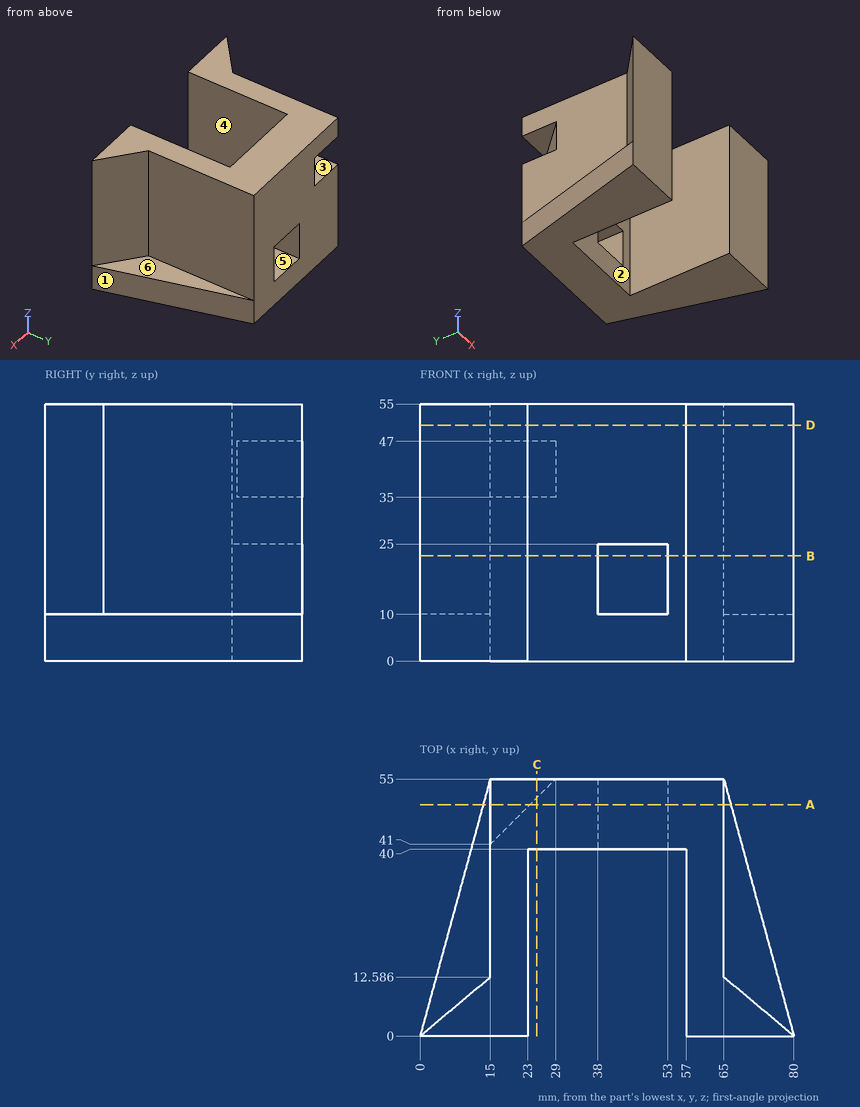
Design review of the part shown in the three views and the two pictorial views. Dimensions are in mm from the part's minimum x, y and z. A direction names the side the tool comes from. Give positions to 0.01 mm unless a question says otherwise; leave off trailing zeros. Loops run counter-clockwise (first coordinate to the right, second up) from the corner with the lowest first, then second, coordinate; pieces in that order, holes last. Notation, with made-up numbers: (61, -28) -> (116, -28) arc R17 cw to (116, -10) -> close; hole circle Ø3 at (78, 22.25). An arc over 180 degrees is marked (long way). Write each question's results on one line, items separated by ' | '.
1) Take a section at D-D, the plane z = 50.5. Give the boundary of the cut face in (x, y), plus the area to 3 significant figures.
Conclusion:
outline: (0, 0) -> (23, 0) -> (23, 40) -> (57, 40) -> (57, 0) -> (80, 0) -> (65, 12.59) -> (65, 55) -> (15, 55) -> (15, 12.59) -> close | area: 1,580 mm^2
2) Take a section at B-B, the plane z = 22.5. Give the boundary of the cut face in (x, y).
Conclusion:
outline: (0, 0) -> (23, 0) -> (23, 40) -> (38, 40) -> (38, 55) -> (15, 55) -> (15, 12.59) -> close; (53, 40) -> (57, 40) -> (57, 0) -> (80, 0) -> (65, 12.59) -> (65, 55) -> (53, 55) -> close
3) Draft analysis for pull direction X (two halves, no side actions). For the marked faces 1, 2 and 3, state which applies: pulls with the +X half, pulls with the -X half, needs draft (parallel to the pull), parting line crosses it, or undercut.
Conclusion:
face 1: pulls with the +X half | face 2: undercut | face 3: needs draft
4) For line 1 along X through (y, z) = (52, 16); line 2 along X through (y, z) = (16, 49.5); line 3 along Z through (x, y) = (12, 24), list the stretches that pass through material, from the lowest coordinate up. Write a range as from..to.
Conclusion:
line 1: x = 15..38, 53..65 | line 2: x = 15..23, 57..65 | line 3: z = 0..10
5) Tool access review of the marked faces 4, 5 and 6: name each direction out of +Z, -Z, +X, -X, +Y, -Y from which nothing blocks a thin tool from reaching the whole face with its end or side.
Conclusion:
face 4: +Z, -Z, -Y | face 5: +Y, -Y | face 6: +Z, +X, +Y
6) Insertion check: pin 1 Ø21 at (y, z) = (44, 28.5) entering from -X; pin 2 Ø1 at (y, z) = (32, 42.5) entering from +X; pin 3 Ø1 at (y, z) = (10.5, 22.5) entering from +X. Each pin has a flat end and moves straight along its axis. Give the tip position at first contact, or say it passes through.
Conclusion:
pin 1: stops at x = 15 | pin 2: stops at x = 65 | pin 3: stops at x = 68.08
7) Take a section at A-A, the plane y = 49.5. Give the boundary of the cut face in (x, z).
Conclusion:
outline: (13.5, 0) -> (66.5, 0) -> (66.5, 10) -> (65, 10) -> (65, 55) -> (15, 55) -> (15, 47) -> (23.5, 47) -> (23.5, 35) -> (15, 35) -> (15, 10) -> (13.5, 10) -> close; hole (38, 10) -> (53, 10) -> (53, 25) -> (38, 25) -> close
8) Take a section at C-C, the plane x = 25. Give the boundary of the cut face in (y, z).
Conclusion:
outline: (40, 0) -> (55, 0) -> (55, 35) -> (51, 35) -> (51, 47) -> (55, 47) -> (55, 55) -> (40, 55) -> close
